Here's how the part is built. I have some questions about the finished solid (model axes, mm). Face numbers are marked on the shaded views. A direction names the side the tool comes from. Give positions to 0.01 mm unless a question says otherwise; leave off trailing zeros. Write each loop counter-clockwise with the first axis right and the second up, starting at its lowest first coordinate (ties: lowest second). Pieces come first, ordered by that corner, then holes. Notation, with made-up numbers: (-1, -11.5) - (24, -11.5) arc R7 cw to (24, -4.5) - close; hole circle Ø8 at (-2, 38.25). An arc over 180 degrees is marked (long way). One line per item, written item: value. Start each with the question number.
1) Please list where these lines run through material, in increasing order: L1, parallel to Z at x = 0.75, y = 27.5; L2, parallel to X at y = 32.5, z = 43; L3, parallel to Y at x = -2.75, z = 9. Write a range as [from, to].
2) Imagine slicing it at C-C on z = 58. Write out the boundary of the cut face in (x, y).
3) Imagine slicing it at D-D on x = -12. Write out the boundary of the cut face in (y, z).
4) Imagine slicing it at A-A on y = 28. Write out the boundary of the cut face in (x, z).
5) Imagine slicing it at B-B on x = -5. Write out the boundary of the cut face in (y, z).
6) On a 3-axis mill with a long thin cutter (end or side, diameter ignored), from which of +Z, -Z, +X, -X, +Y, -Y can I reach the whole of each face in a straight line? I mean the marked faces 1 and 2. Say none if no direction works.
7) I'm going to push flat-ended pins straight in: P1, Ø1, axis at x = -5.5, z = 53, coming from the +Y side; P2, Ø6, axis at y = 30.5, z = 15, coming from the +X side; P3, Ø1, axis at y = 25, z = 22.5, coming from the -X side. Where does each tip first touch, or does it pass through?
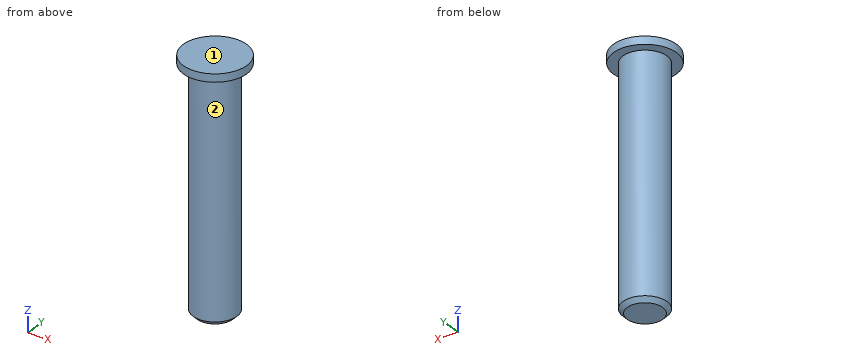
from build123d import *

# Parameters (mm, degrees)
SKETCH_1_R      = 6
EXTRUDE_1_DEPTH = 40
SKETCH_1_4_R    = 6
EXTRUDE_3_DEPTH = 60
SKETCH_2_R      = 8
EXTRUDE_4_DEPTH = 2


# Read off the part's stored shape, not the designer's step: 7/16-14 机械螺纹 螺柱1
with BuildPart() as part:
    # 草图1 → 凸台-拉伸1 (new body)
    with BuildSketch(Plane.XY):
        with Locations((-5, 28)):
            Circle(SKETCH_1_R)
    extrude(amount=EXTRUDE_1_DEPTH)

    # 草图1<4> → 凸台-拉伸3 (add)
    with BuildSketch(Plane.XY):
        with Locations((-5, 28)):
            Circle(SKETCH_1_4_R)
    extrude(amount=EXTRUDE_3_DEPTH)

    # 草图2 → 凸台-拉伸4 (add)
    with BuildSketch(Plane.XY.offset(60)):
        with Locations((-5, 28)):
            Circle(SKETCH_2_R)
    extrude(amount=EXTRUDE_4_DEPTH)

    # 7/16-14 机械螺纹 螺柱1 outline → 7/16-14 机械螺纹 螺柱1 (revolve, cut)
    with BuildSketch(Plane(origin=(-5, 28, 0), x_dir=(1, 0, 0), z_dir=(0, -1, 0))):
        Polygon((4.47675, 0), (6, 0), (6, 60), (5.55625, 60), (5.55625, 1.0795), align=None)
    revolve(axis=Axis((-5, 28, 0), (0, 0, 1)), mode=Mode.SUBTRACT)


solid = part.part
Numbers:
1. L1: [60, 62]
1. L2: [-8.26, -1.74]
1. L3: [22.92, 33.08]
2. outline: circle Ø11.11 at (-5, 28)
3. outline: (24.13, 60) - (31.87, 60) - (31.87, 62) - (24.13, 62) - close
4. outline: (-13, 60) - (-10.56, 60) - (-10.56, 1.08) - (-9.48, 0) - (-0.52, 0) - (0.56, 1.08) - (0.56, 60) - (3, 60) - (3, 62) - (-13, 62) - close
5. outline: (20, 60) - (22.44, 60) - (22.44, 1.08) - (23.52, 0) - (32.48, 0) - (33.56, 1.08) - (33.56, 60) - (36, 60) - (36, 62) - (20, 62) - close
6. face 1: +Z, +X, -X, +Y, -Y
6. face 2: -Z
7. P1: y = 33.56
7. P2: x = 0.56
7. P3: x = -9.96
